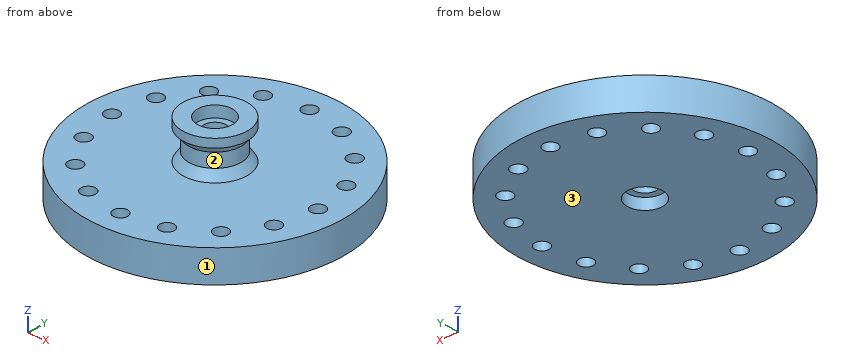
from build123d import *

# Parameters (mm, degrees)
F0_W     = 11
F0_H     = 7
F2_R     = 11
F3_DEPTH = 7
F4_R     = 7
F5_DEPTH = 80
F6_R     = 4.5
F7_DEPTH = 41.7


with BuildPart() as f1:
    # F0 (on Front) → F1 (revolve)
    with BuildSketch(Plane.XZ):
        Polygon((-20, 20), (-80, 20), (-80, 0), (-11, 0), (-11, 7), (0, 7), (0, 20), (0, 37), (-10.908018, 37), (-10.908018, 44), (-20, 44.023235), (-20, 38.700003), (-16.150784, 34.302171), (-16.150784, 25.613375), align=None)
        with Locations((-5.5, 3.5)):
            Rectangle(F0_W, F0_H)
    revolve(axis=Axis((0, 0, 77.767195), (0, 0, -1)))

    # F2 (on face) → F3 (cut)
    with BuildSketch(Plane(origin=(0, 0, 0), x_dir=(1, 0, 0), z_dir=(0, 0, -1))):
        Circle(F2_R)
    extrude(amount=-F3_DEPTH, mode=Mode.SUBTRACT)

    # F4 (on face) → F5 (cut)
    with BuildSketch(Plane(origin=(0, 0, 7), x_dir=(1, 0, 0), z_dir=(0, 0, -1))):
        Circle(F4_R)
    extrude(amount=-F5_DEPTH, mode=Mode.SUBTRACT)

    # F6 (on face) → F7 (cut)
    with BuildSketch(Plane.XY.offset(20)):
        with Locations((-45.961941, 45.961941)):
            Circle(F6_R)
        with Locations((-24.874423, 60.05217)):
            Circle(F6_R)
        with Locations((0, 65)):
            Circle(F6_R)
        with Locations((24.874423, 60.05217)):
            Circle(F6_R)
        with Locations((45.961941, 45.961941)):
            Circle(F6_R)
        with Locations((60.05217, 24.874423)):
            Circle(F6_R)
        with Locations((65, 0)):
            Circle(F6_R)
        with Locations((60.05217, -24.874423)):
            Circle(F6_R)
        with Locations((45.961941, -45.961941)):
            Circle(F6_R)
        with Locations((24.874423, -60.05217)):
            Circle(F6_R)
        with Locations((0, -65)):
            Circle(F6_R)
        with Locations((-24.874423, -60.05217)):
            Circle(F6_R)
        with Locations((-45.961941, -45.961941)):
            Circle(F6_R)
        with Locations((-60.05217, -24.874423)):
            Circle(F6_R)
        with Locations((-65, 0)):
            Circle(F6_R)
        with Locations((-60.05217, 24.874423)):
            Circle(F6_R)
    extrude(amount=-F7_DEPTH, mode=Mode.SUBTRACT)


solid = f1.part
Design review of the part built by this model. Coordinates are the model's own, in mm. Face numbers are marked on the shaded views. Round coordinates to 2 decimals unless told otherwise and drop trailing zeros. Write each loop counter-clockwise with the first axis right and the second up, starting at its lowest first coordinate (ties: lowest second). Pieces come first, ordered by that corner, then holes.
Item 1: Consider section A-A on x = 0. Count the separate pieces of the cut face and the enclosed holes in it, and give its area (3 significant figures).
Item 2: Wall thickness on L1, parallel to Y at x = 0, z = 15.25; L2, parallel to X at y = 50, z = 6; L3, parallel to Z at x = -28, y = 64: over which ranges is each line inside the solid? List them lowest first.
Item 3: Consider section C-C on x = -27. Give the boundary of the cut face in (y, z), and give its area (3 significant figures).
Item 4: Consider section D-D on z = 30. Give the boundary of the cut face in (x, y).
Item 5: For pin 1 Ø1.5 at (x, z) = (-50.5, 12.5) entering from -Y; pin 2 Ø12 at (x, z) = (-17.5, 37.5) entering from -Y; pin 3 Ø6.5 at (x, y) = (-4, 2) entering from +Z; pin 4 Ø5.5 at (x, y) = (-45.96, -45.96) entering from +Z, all flat-tipped, find the tip position at first contact; note any pin that passes through.
Item 6: Draft analysis for pull direction Z (two halves, no side actions). For the marked faces 1, 2 and 3, state which applies: released by +Z, released by -Z, zero draft, split by the parting line, or undercut.
Check values:
1. separate pieces: 4
1. enclosed holes: 0
1. area: 2,970 mm2
2. L1: y = -80 to -69.5, -60.5 to -7, 7 to 60.5, 69.5 to 80
2. L2: x = -62.45 to -47.95, -43.98 to 43.98, 47.95 to 62.45
2. L3: z = 0 to 20
3. outline: (-75.31, 0) - (-64.02, 0) - (-64.02, 20) - (-75.31, 20) - close; (-56.09, 0) - (56.09, 0) - (56.09, 20) - (-56.09, 20) - close; (64.02, 0) - (75.31, 0) - (75.31, 20) - (64.02, 20) - close
3. area: 2,690 mm2
4. outline: circle Ø32.3 at (0, 0); hole circle Ø14 at (0, 0)
5. pin 1: stops at y = -62.65
5. pin 2: stops at y = -16.28
5. pin 3: stops at z = 37
5. pin 4: passes through
6. face 1: zero draft
6. face 2: undercut
6. face 3: released by -Z
